Can you work these out from the model? Positions are in its coordinate system, mm. A direction names the side the tool comes from. Coordinates: 2 decimals unless noted, no trailing zeros. Order: outer loops, then holes, each group sorted by start corner. A loop starts at its lowest first (then second) coordinate and runs counter-clockwise, first axis right, second up. Notation, with made-up numbers: (2.25, 61) -> (39.25, 61) arc R16 ccw to (39.25, 70) -> close; hole circle Ø7 at (21.5, 1.25). An arc over 180 degrees is marked (long way). Write item = value, one per line.
Autodesk Fusion 360 part; units mm, degrees
sketch "Base" plane through (0, 0, 0) normal (0, 0, 1) x (1, 0, 0)
  circle A0 centre (0, 0) radius 40
  circle A1 centre (0, 0) radius 4.3
  line L0 (0, 0) -> (50, 0) construction
  circle A2 centre (25, 0) radius 1.75
  line L1 (0, 0) -> (0, 40) construction
  circle A3 centre (-25, 0) radius 1.75
  circle A4 centre (50, 0) radius 3.2
  circle A5 centre (0, 0) radius 10
  line L2 (7.0711, -7.0711) -> (28.2843, -28.2843)
  line L3 (7.0711, -7.0711) -> (0, 0) construction
  line L4 (7.0711, 7.0711) -> (3.0406, 3.0406)
  line L5 (7.0711, -7.0711) -> (3.0406, -3.0406)
  line L6 (7.0711, 7.0711) -> (28.2843, 28.2843)
  circle A6 centre (50, 0) radius 7
  line L7 (49.02, 6.9311) -> (39.6061, 5.6)
  line L8 (39.6061, 5.6) -> (0, 0) construction
  line L9 (49.02, -6.9311) -> (39.6061, -5.6)
  circle A7 centre (50, 0) radius 5.5
  dimension "d1" = 80
  dimension "d4" = 8.6
  dimension "d8" = 25
  dimension "d9" = 3.5
  dimension "d13" = 6.4
  dimension "d21" = 20
  dimension "d49" = 14
  dimension "d50" = 45
  dimension "d51" = 50
  dimension "d52" = 11
extrude "Extrude1" add sketch "Base" against normal blind 13 contours A0 A5 L2 L6 | A0 A6 L7 L9 | A6 | A2 | A7 picked at (21.3272, -10.7092) makes body 1
extrude "Extrude6" add sketch "Base" against normal blind 3 contours A1 A5 L4 L5 picked at (8.0592, -0.6222) bodies 1
extrude "Extrude7" cut sketch "Base" against normal blind 6 contours A7 bodies 1
pattern_circular "C-Pattern2" count 4 over 360 about axis through (0, 0, 1.75) along (0, 0, 1) of bodies 1 makes body 2 at (0.1023, 27.8337, 0) makes body 3 at (-27.8337, 0.1023, 0) makes body 4 at (-0.1023, -27.8337, 0)
extrude "Extrude5" add sketch "Base" along normal blind 4 separate body contours A2 | A3 makes body 5 at (26.7478, -0.0872, 2.6667) makes body 6 at (-23.2522, -0.0872, 2.6667)
combine "Combine1" operation add target body 1 tool bodies 6 5 2 3 4
copy_body "Body->Comp1" bodies 1 removing the originals makes body 7 in component "Mirror_Pyramid_Mount"
component "Mirror_Pyramid_Mount" placed x (1, 0, 0) y (0, 1, 0) z (0, 0, 1) at (0, 0, 0)
equation "d51 = ( 2 * 25 ) * 1 mm"
Item 1: I want a section at C-C, the plane x = 25. Please give me the cut outline in (y, z), plus the area to 3 significant figures.
A:
outline = (-31.22, -13) -> (31.22, -13) -> (31.22, 0) -> (1.75, 0) -> (1.75, 4) -> (-1.75, 4) -> (-1.75, 0) -> (-31.22, 0) -> close
area = 826 mm2
Item 2: If we mould it in two halves opening along Y, with no side actions, what happens to faces 4 (the flat face through (-44.379, 6.275, -6.409)), 5 (the cylindrical face through (-44.505, -0.242, -2.958)), 6 (the cylindrical face through (57, 0, -6)), 7 (the flat face through (-1, -12, 0))? For each: pulls with the +Y half, pulls with the -Y half, needs draft (parallel to the pull), parting line crosses it, or undercut.
A:
face_4 = pulls with the +Y half
face_5 = undercut
face_6 = parting line crosses it
face_7 = needs draft
Item 3: For faces 1 (the cylindrical face through (0.242, -44.505, -2.958)), 2 (the flat face through (6.275, -44.379, -6.409)), 3 (the cylindrical face through (-5.37, 8.436, -7.93)), which set-ups out of +Z, -Z, +X, -X, +Y, -Y let a thin tool reach every point of the face, with its end or its side?
A:
face_1 = +Z
face_2 = +Z, -Z, +X
face_3 = -Z
Item 4: If I drill on probe 1 along Y at (x, z) = (50, -3.3); probe 2 along Y at (x, z) = (50, -9.5), over which ranges is the centre line in solid material (lowest first)?
A:
probe_1 = -7 to -5.5, 5.5 to 7
probe_2 = -7 to -3.2, 3.2 to 7
Item 5: I'm going to push flat-ended pins straight in: P1, Ø12, axis at x = 49.5, y = 1.5, coming from the +Z side; P2, Ø10, axis at x = 0, y = 50, coming from the +Z side; P3, Ø10, axis at x = -39, z = -6, coming from the -Y side. Where does each tip first touch, or does it pass through?
A:
P1 = 0
P2 = -6
P3 = -21.07
Item 6: I want a section at B-B, the plane y = 0. Give the number of separate pieces and of enclosed holes in the cut face, plus the area to 3 significant figures.
A:
separate_pieces = 4
enclosed_holes = 0
area = 1,060 mm2
Item 7: I want a section at A-A, the plane z = -11.5. Please give me the cut outline in (x, y), plus the area to 3 significant figures.
A:
outline = (-49.02, -6.93) -> (-39.61, -5.6) arc R40 ccw to (-5.6, -39.61) -> (-6.93, -49.02) arc R7 ccw (long way) to (6.93, -49.02) -> (5.6, -39.61) arc R40 ccw to (39.61, -5.6) -> (49.02, -6.93) arc R7 ccw (long way) to (49.02, 6.93) -> (39.61, 5.6) arc R40 ccw to (5.6, 39.61) -> (6.93, 49.02) arc R7 ccw (long way) to (-6.93, 49.02) -> (-5.6, 39.61) arc R40 ccw to (-39.61, 5.6) -> (-49.02, 6.93) arc R7 ccw (long way) to start; hole circle Ø6.4 at (-50, 0); hole circle Ø20 at (0, 0); hole circle Ø6.4 at (0, -50); hole circle Ø6.4 at (0, 50); hole circle Ø6.4 at (50, 0)
area = 5,410 mm2
Item 8: I want a section at D-D, the plane y = 27. Please give me the cut outline in (x, z), plus the area to 3 significant figures.
A:
outline = (-29.51, -13) -> (29.51, -13) -> (29.51, 0) -> (-29.51, 0) -> close
area = 767 mm2
